```python
from build123d import *

# Parameters (mm, degrees)
F0_R     = 54.2445542545
F1_DEPTH = 38.354
F2_R     = 26.4064404113
F3_DEPTH = 23.114
F4_T     = -2.54


with BuildPart() as f1:
    # F0 (on Top) → F1 (new body)
    with BuildSketch(Plane.XY):
        Circle(F0_R)
    extrude(amount=-F1_DEPTH)

    # F2 (on face) → F3 (join)
    with BuildSketch(Plane(origin=(0, 0, -38.354), x_dir=(1, 0, 0), z_dir=(0, 0, -1))):
        Circle(F2_R)
    extrude(amount=F3_DEPTH)

    # F4
    f4_openings = [f1.faces().sort_by_distance(p)[0] for p in [
        (0, 0, -61.468),
    ]]
    offset(amount=F4_T, openings=f4_openings, kind=Kind.INTERSECTION)


solid = f1.part
```
Geometry: final body of the model. Coordinates: model frame, mm. A direction names the side the tool comes from. Round coordinates to 2 decimals unless told otherwise and drop trailing zeros. Order: outer loops, then holes, each group sorted by start corner. A loop starts at its lowest first (then second) coordinate and runs counter-clockwise, first axis right, second up. Notation, with made-up numbers: M 37.25,44 L 80.25,44 A21 ccw 80.25,65 Z; hole C -0.5,56.25 d4. An arc over 180 degrees is marked long. One line per item, written item: value.
(1) Cut plane D-D (x = -47). Return the cut outline in (y, z).
Result sheet:
outline: M -27.08,-38.35 L 27.08,-38.35 L 27.08,0 L -27.08,0 Z; hole M -21.55,-35.81 L 21.55,-35.81 L 21.55,-2.54 L -21.55,-2.54 Z
(2) Reachability of faces 1 (the flat face through (23.3, 12.8, -38.354)), 2 (the cylindrical face through (51.74, 16.29, -18.91)), 3 (the flat face through (22, -11, -35.814)) from +Z, -Z, +X, -X, +Y, -Y: full face, straight path, thin tool, end or side. Return the list, or none.
Result sheet:
face 1: -Z
face 2: +Z, -Z
face 3: none
(3) Cut plane A-A (y = 0). Return the cut outline in (x, z), and give its area (3 significant figures).
Result sheet:
outline: M -54.24,-38.35 L -26.41,-38.35 L -26.41,-61.47 L -23.87,-61.47 L -23.87,-35.81 L -51.7,-35.81 L -51.7,-2.54 L 51.7,-2.54 L 51.7,-35.81 L 23.87,-35.81 L 23.87,-61.47 L 26.41,-61.47 L 26.41,-38.35 L 54.24,-38.35 L 54.24,0 L -54.24,0 Z
area: 716 mm2
(4) Cut plane C-C (y = -30.5). Return the cut outline in (x, z).
Result sheet:
outline: M -44.86,-38.35 L 44.86,-38.35 L 44.86,0 L -44.86,0 Z; hole M -41.75,-35.81 L 41.75,-35.81 L 41.75,-2.54 L -41.75,-2.54 Z
(5) Line query: probe 1 along Z at (x, y) = (40, -9); probe 2 along Z at (x, y) = (-24, 10.5); probe 3 along Y at (x, z) = (0, -10). Output: solid intervals per line, ascending. Write a range as [from, to].
Result sheet:
probe 1: [-38.35, -35.81], [-2.54, 0]
probe 2: [-61.47, -35.81], [-2.54, 0]
probe 3: [-54.24, -51.7], [51.7, 54.24]
(6) Pin query (flat end, axial travel): P1, Ø12, axis at x = 4.5, z = -30, coming from the +Y side; P2, Ø5, axis at x = -8, z = -49.5, coming from the -Y side; P3, Ø1.5, axis at y = 31.5, z = -38.5, coming from the +X side. Return the tip coordinate at first contact, or that it passes through.
Result sheet:
P1: y = 54.24
P2: y = -25.83
P3: x = 44.68
(7) Pull-direction query (X, two-part tool) for faces 4 (the cylindrical face through (49.317, 15.531, -18.944)), 5 (the flat face through (-1, 1, 0)), 6 (the cylindrical face through (-20.955, 16.068, -49.749)), 7 (the cylindrical face through (-18.94, 14.52, -48.46)); classes: pulls with the +X half, pulls with the -X half, needs draft (parallel to the pull), parting line crosses it, or undercut.
Result sheet:
face 4: undercut
face 5: needs draft
face 6: parting line crosses it
face 7: undercut
